Part model, mm, in its own coordinate system. A direction names the side the tool comes from. Give positions to 0.01 mm unless a question says otherwise; leave off trailing zeros. Write each loop counter-clockwise with the first axis right and the second up, starting at its lowest first coordinate (ties: lowest second). Pieces come first, ordered by that corner, then holes. Notation, with made-up numbers: M 25.5,1 L 76.5,1 A27 ccw 76.5,26 Z; hole C 58,65 d5. An arc over 180 degrees is marked long. Use CSV: the item, a comma, the result in double quotes. Start each with the question number.
Item 1: Pin check, flat tips, straight feed: pin 1 (1.5 mm diameter, centred on y = 2, z = -54, fed in from +X); pin 2 (1 mm diameter, centred on x = 44.5, z = -65.5, fed in from -Y); pin 3 (4 mm diameter, centred on y = 52.5, z = -66.5, fed in from +X). Stop position of each tip, or through.
Item 2: Cut at C-C (z = -96.5). List the corners of the cut face in (x, y), then the cut area to 3 significant figures.
Item 3: Drill centre lines: line 1 (Z direction, x = 0, y = 26); line 2 (Y direction, x = -5.5, z = -46.5); line 3 (Y direction, x = 45.5, z = -79.5). Where is each one in solid material? Low to high. Write a range as [from, to].
Item 4: Cut at D-D (y = 21.5). List the corners of the cut face in (x, z).
Item 5: Cut at B-B (y = 6.5). List the corners of the cut face in (x, z).
Item 6: Mould opens along Z. For faces 6 (the flat face through (50, 3, -56)), 7 (the flat face through (-10, 77, -88)) say: released by +Z, released by -Z, zero draft, split by the parting line, or undercut.
Item 7: Which spindle directions (+Z, -Z, +X, -X, +Y, -Y) get a long thin tool onto all of the face, cutting with end or side? Do faces 1 (the flat face through (-72.7, 19, -93.2)), 2 (the flat face through (73.3, 19, -37.2)), 3 (the flat face through (-44, 16, -82)), 4 (the flat face through (-73, 11, -21)), 5 (the flat face through (-12, 66, -28)). Say none if no direction does.
Item 8: Cut at A-A (x = -73). List the corners of the cut face in (y, z).
from build123d import *

# Parameters (mm, degrees)
BOSS_EXTRUDE1_DEPTH = 114
SKETCH3_W           = 82.5
SKETCH3_H           = 94
CUT_EXTRUDE1_DEPTH  = 3
CUT_EXTRUDE2_DEPTH  = 17
SKETCH5_R           = 19
BOSS_EXTRUDE2_DEPTH = 3
SKETCH6_R           = 47.5
SKETCH6_R_2         = 31
BOSS_EXTRUDE4_DEPTH = 61
SKETCH8_W           = 3
SKETCH8_H           = 35.544994967
SKETCH9_R           = 1.5
CUT_EXTRUDE3_DEPTH  = 5


with BuildPart() as part:
    # Sketch2 → Boss-Extrude1 (new body)
    with BuildSketch(Plane.XY):
        Polygon((-102, 0), (-97, 16), (97, 16), (102, 0), align=None)
    extrude(amount=-BOSS_EXTRUDE1_DEPTH)

    # Sketch3 → Cut-Extrude1 (cut)
    with BuildSketch(Plane.XZ):
        with Locations((-50.75, -57)):
            Rectangle(SKETCH3_W, SKETCH3_H)
        with Locations((50.75, -57)):
            Rectangle(SKETCH3_W, SKETCH3_H)
    extrude(amount=-CUT_EXTRUDE1_DEPTH, mode=Mode.SUBTRACT)

    # Sketch4 → Cut-Extrude2 (cut, through all)
    with BuildSketch(Plane(origin=(0, 16, 0), x_dir=(1, 0, 0), z_dir=(0, 1, 0))):
        with BuildLine():
            Line((-76, 77), (-70, 77))
            ThreePointArc((-70, 77), (-62, 85), (-70, 93))
            Line((-70, 93), (-76, 93))
            ThreePointArc((-76, 93), (-84, 85), (-76, 77))
        make_face()
        with BuildLine():
            ThreePointArc((70, 77), (62, 85), (70, 93))
            Line((70, 93), (76, 93))
            ThreePointArc((76, 93), (84, 85), (76, 77))
            Line((76, 77), (70, 77))
        make_face()
        with BuildLine():
            ThreePointArc((-70, 37), (-62, 29), (-70, 21))
            Line((-70, 21), (-76, 21))
            ThreePointArc((-76, 21), (-84, 29), (-76, 37))
            Line((-76, 37), (-70, 37))
        make_face()
        with BuildLine():
            Line((76, 37), (70, 37))
            ThreePointArc((70, 37), (62, 29), (70, 21))
            Line((70, 21), (76, 21))
            ThreePointArc((76, 21), (84, 29), (76, 37))
        make_face()
    extrude(amount=-CUT_EXTRUDE2_DEPTH, mode=Mode.SUBTRACT)

    # Sketch5 → Boss-Extrude2 (add)
    with BuildSketch(Plane(origin=(0, 16, 0), x_dir=(1, 0, 0), z_dir=(0, 1, 0))):
        with Locations(Location((-73, 85, 0), (0, 0, 180))):  # turned: the seam where the file's is
            Circle(SKETCH5_R)
        with BuildLine():
            ThreePointArc((-70, 93), (-62, 85), (-70, 77))
            Line((-70, 77), (-76, 77))
            ThreePointArc((-76, 77), (-84, 85), (-76, 93))
            Line((-76, 93), (-70, 93))
        make_face(mode=Mode.SUBTRACT)
        with Locations(Location((73, 85, 0), (0, 0, 180))):  # turned: the seam where the file's is
            Circle(SKETCH5_R)
        with BuildLine():
            ThreePointArc((76, 93), (84, 85), (76, 77))
            Line((76, 77), (70, 77))
            ThreePointArc((70, 77), (62, 85), (70, 93))
            Line((70, 93), (76, 93))
        make_face(mode=Mode.SUBTRACT)
        with Locations(Location((73, 29, 0), (0, 0, 180))):  # turned: the seam where the file's is
            Circle(SKETCH5_R)
        with BuildLine():
            ThreePointArc((70, 21), (62, 29), (70, 37))
            Line((70, 37), (76, 37))
            ThreePointArc((76, 37), (84, 29), (76, 21))
            Line((76, 21), (70, 21))
        make_face(mode=Mode.SUBTRACT)
        with Locations(Location((-73, 29, 0), (0, 0, 180))):  # turned: the seam where the file's is
            Circle(SKETCH5_R)
        with BuildLine():
            ThreePointArc((-76, 21), (-84, 29), (-76, 37))
            Line((-76, 37), (-70, 37))
            ThreePointArc((-70, 37), (-62, 29), (-70, 21))
            Line((-70, 21), (-76, 21))
        make_face(mode=Mode.SUBTRACT)
    extrude(amount=BOSS_EXTRUDE2_DEPTH)

    # Sketch6 → Boss-Extrude4 (add)
    with BuildSketch(Plane(origin=(0, 16, 0), x_dir=(1, 0, 0), z_dir=(0, 1, 0))):
        with Locations(Location((0, 57, 0), (0, 0, 180))):  # turned: the seam where the file's is
            Circle(SKETCH6_R)
        with Locations(Location((0, 57, 0), (0, 0, 180))):  # turned: the seam where the file's is
            Circle(SKETCH6_R_2, mode=Mode.SUBTRACT)
    extrude(amount=BOSS_EXTRUDE4_DEPTH)

    # Sketch8 → Cut-Revolve1 (revolve, cut)
    with BuildSketch(Plane.XY.offset(-57)):
        with Locations((-31, 48.227502517)):
            Rectangle(SKETCH8_W, SKETCH8_H)
    revolve(axis=Axis((0, 107.106199385, -57), (0, -1, 0)), mode=Mode.SUBTRACT)

    # Sketch9 → Cut-Extrude3 (cut)
    with BuildSketch(Plane(origin=(0, 16, 0), x_dir=(1, 0, 0), z_dir=(0, 1, 0))):
        with Locations(Location((-23.5, 57, 0), (0, 0, 180))):  # turned: the seam where the file's is
            Circle(SKETCH9_R)
    extrude(amount=-CUT_EXTRUDE3_DEPTH, mode=Mode.SUBTRACT)


solid = part.part
Worked answers:
1,pin 1,"stops at x = 101.61"
1,pin 2,"stops at y = 3"
1,pin 3,"stops at x = 46.9"
2,outline,"M -102,0 L -92,0 L -92,3 L -9.5,3 L -9.5,0 L 9.5,0 L 9.5,3 L 92,3 L 92,0 L 102,0 L 97,16 L 88.12,16 L 88.12,19 L 57.88,19 L 57.88,16 L 26.38,16 L 26.38,77 L -26.38,77 L -26.38,16 L -57.88,16 L -57.88,19 L -88.12,19 L -88.12,16 L -97,16 Z"
2,area,"6,090 mm^2"
3,line 1,"z = [-104.5, -88], [-26, -9.5]"
3,line 2,"y = [0, 16]"
3,line 3,"y = [3, 16]"
4,outline,"C 0,-57 d95; hole C 0,-57 d62"
5,outline,"M -99.97,-114 L 99.97,-114 L 99.97,0 L -99.97,0 Z; hole M -76,-93 L -70,-93 A8 ccw -70,-77 L -76,-77 A8 ccw Z; hole M -76,-37 L -70,-37 A8 ccw -70,-21 L -76,-21 A8 ccw Z; hole M 70,-93 L 76,-93 A8 ccw 76,-77 L 70,-77 A8 ccw Z; hole M 70,-37 L 76,-37 A8 ccw 76,-21 L 70,-21 A8 ccw Z"
6,face 6,"undercut"
6,face 7,"zero draft"
7,face 1,"+Z, -Z, -X, +Y"
7,face 2,"+Z, -Z, +X, +Y"
7,face 3,"+Y"
7,face 4,"+Y, -Y"
7,face 5,"none"
8,outline,"M 0,-114 L 16,-114 L 16,-104 L 19,-104 L 19,-93 L 3,-93 L 3,-104 L 0,-104 Z; M 0,-10 L 3,-10 L 3,-21 L 19,-21 L 19,-10 L 16,-10 L 16,0 L 0,0 Z; M 3,-77 L 19,-77 L 19,-66 L 16,-66 L 16,-48 L 19,-48 L 19,-37 L 3,-37 Z"
